from build123d import *

# Parameters (mm, degrees)
BOSS_EXTRUDE1_START = 80.3
BOSS_EXTRUDE1_DEPTH = 2.4
BOSS_EXTRUDE2_START = 80.3
BOSS_EXTRUDE2_DEPTH = 1.6
BOSS_EXTRUDE3_START = 79.3
BOSS_EXTRUDE3_DEPTH = 4.4
BOSS_EXTRUDE4_START = 79.3
SKETCH4_R           = 2.6
BOSS_EXTRUDE4_DEPTH = 4.4
BOSS_EXTRUDE5_START = 82.1
BOSS_EXTRUDE5_DEPTH = 1.6
CHAMFER1_SIZE       = 0.5


with BuildPart() as part:
    # Sketch1 → Boss-Extrude1 (new body)
    with BuildSketch(Plane.XY.offset(BOSS_EXTRUDE1_START)):
        with BuildLine():
            Line((-6, 29), (6, 29))
            ThreePointArc((6, 29), (9.535533906, 30.464466094), (11, 34))
            Line((11, 34), (11, 45))
            ThreePointArc((11, 45), (9.535533906, 48.535533906), (6, 50))
            Line((6, 50), (-6, 50))
            ThreePointArc((-6, 50), (-9.535533906, 48.535533906), (-11, 45))
            Line((-11, 45), (-11, 34))
            ThreePointArc((-11, 34), (-9.535533906, 30.464466094), (-6, 29))
        make_face()
    extrude(amount=BOSS_EXTRUDE1_DEPTH)

    # Sketch2 → Boss-Extrude2 (add)
    with BuildSketch(Plane.XY.offset(BOSS_EXTRUDE2_START)):
        with BuildLine():
            Line((4.5, 53.5), (4.5, 54.7))
            ThreePointArc((4.5, 54.7), (3.181980515, 57.881980515), (0, 59.2))
            ThreePointArc((0, 59.2), (-3.181980515, 57.881980515), (-4.5, 54.7))
            Line((-4.5, 54.7), (-4.5, 53.5))
            ThreePointArc((-4.5, 53.5), (-3.181980515, 50.318019485), (0, 49))
            ThreePointArc((0, 49), (3.181980515, 50.318019485), (4.5, 53.5))
        make_face()
    extrude(amount=BOSS_EXTRUDE2_DEPTH)


with BuildPart() as body_2:
    # Sketch3 → Boss-Extrude3 (new body)
    with BuildSketch(Plane.XY.offset(BOSS_EXTRUDE3_START)):
        with BuildLine():
            Line((-1.8, 56), (-1.8, 53.6))
            ThreePointArc((-1.8, 53.6), (0, 51.8), (1.8, 53.6))
            Line((1.8, 53.6), (1.8, 56))
            ThreePointArc((1.8, 56), (0, 57.8), (-1.8, 56))
        make_face()
    extrude(amount=BOSS_EXTRUDE3_DEPTH)


with BuildPart() as part_1:
    add(part.part)

    # Combine1: cut body 2
    add(body_2.part, mode=Mode.SUBTRACT)


with BuildPart() as body_2_2:
    # Sketch4 → Boss-Extrude4 (new body)
    with BuildSketch(Plane.XY.offset(BOSS_EXTRUDE4_START)):
        with Locations((0, 53.6)):
            Circle(SKETCH4_R)
    extrude(amount=BOSS_EXTRUDE4_DEPTH)


with BuildPart() as part_2:
    add(part_1.part)

    # Combine2: cut body 2 2
    add(body_2_2.part, mode=Mode.SUBTRACT)


with BuildPart() as body_2_3:
    # Sketch5 → Boss-Extrude5 (new body)
    with BuildSketch(Plane.XY.offset(BOSS_EXTRUDE5_START)):
        with BuildLine():
            Line((-5.5, 31.5), (5.5, 31.5))
            ThreePointArc((5.5, 31.5), (7.621320344, 32.378679656), (8.5, 34.5))
            Line((8.5, 34.5), (8.5, 44.5))
            ThreePointArc((8.5, 44.5), (7.621320344, 46.621320344), (5.5, 47.5))
            Line((5.5, 47.5), (-5.5, 47.5))
            ThreePointArc((-5.5, 47.5), (-7.621320344, 46.621320344), (-8.5, 44.5))
            Line((-8.5, 44.5), (-8.5, 34.5))
            ThreePointArc((-8.5, 34.5), (-7.621320344, 32.378679656), (-5.5, 31.5))
        make_face()
    extrude(amount=BOSS_EXTRUDE5_DEPTH)


with BuildPart() as part_3:
    add(part_2.part)

    # Combine3: cut body 2 3
    add(body_2_3.part, mode=Mode.SUBTRACT)

    # Chamfer1
    chamfer1_edges = [part_3.edges().sort_by_distance(p)[0] for p in [
        (9.535533906, 30.464466094, 82.7),
        (11, 39.5, 82.7),
        (9.535533906, 48.535533906, 82.7),
        (0, 50, 82.7),
        (-9.535533906, 48.535533906, 82.7),
        (-11, 39.5, 82.7),
        (-9.535533906, 30.464466094, 82.7),
        (0, 29, 82.7),
    ]]
    chamfer(chamfer1_edges, length=CHAMFER1_SIZE)


solid = part_3.part
For this review, take the finished solid that the model builds, in its own axes (mm). A direction names the side the tool comes from. Round coordinates to 2 decimals unless told otherwise and drop trailing zeros. Write each loop counter-clockwise with the first axis right and the second up, starting at its lowest first coordinate (ties: lowest second). Pieces come first, ordered by that corner, then holes. Notation, with made-up numbers: (45.5, 30.5) - (104.5, 30.5) arc R24 cw to (104.5, 65.5) - close; hole circle Ø10 at (-2, 86.5). An arc over 180 degrees is marked (long way). Write item = value, one per line. Start each with the question number.
1. For faces 1 (the face through (2, 56, 81.9)), 2 (the face through (7.6, 32.36, 82.4)), 3 (the face through (0, 57.8, 81.1)), list the 3-axis set-ups (+Z, -Z, +X, -X, +Y, -Y) from which the entire face can be reached by the end or side of a thin tool; tool diameter is ignored.
2. Wall thickness on L1, parallel to X at y = 53.6, z = 80.8; L2, parallel to Y at x = 0, z = 80.85; L3, parallel to Y at x = -1, z = 82.15: over which ranges is each line inside the solid? List them lowest first.
3. For pin 1 Ø4 at (x, y) = (5, 41) entering from +Z; pin 2 Ø0.5 at (y, z) = (41.5, 82.5) entering from +X; pin 3 Ø8.5 at (x, y) = (0, 53.6) entering from -Z; pin 4 Ø0.6 at (y, z) = (55.5, 81) entering from +X, all flat-tipped, find the tip position at first contact; note any pin that passes through.
4. Consider section D-D on x = 3.75. State the section outline as (y, z) points.
5. Consider section C-C on x = -2.25. State the section outline as (y, z) points, plus the area to 3 significant figures.
6. Consider section B-B on z = 80.8. State the section outline as (x, y) points.
7. Draft analysis for pull direction Y (two halves, no side actions). For faces 4 (the face through (4.05, 51.54, 81.09)), 5 (the face through (9, 30, 81)), 6 (the face through (-9, 49, 81)), state which applies: released by +Y, released by -Y, zero draft, split by the parting line, or undercut.
8. Consider section A-A on y = 38.5. State the section outline as (x, z) points, plus the area to 4 significant figures.
Evaluation:
q1.face_1 = +Z, +X, -X, +Y
q1.face_2 = +Z
q1.face_3 = +Z, -Z
q2.L1 = -4.5 to -2.6, 2.6 to 4.5
q2.L2 = 29 to 51, 57.8 to 59.2
q2.L3 = 29 to 31.5, 47.5 to 50
q3.pin_1 = 82.1
q3.pin_2 = 10.95
q3.pin_3 = 80.3
q3.pin_4 = 4.47
q4.outline = (29, 80.3) - (50, 80.3) - (50, 82.2) - (49.5, 82.7) - (47.5, 82.7) - (47.5, 82.1) - (31.5, 82.1) - (31.5, 82.7) - (29.5, 82.7) - (29, 82.2) - close; (51.01, 80.3) - (57.19, 80.3) - (57.19, 81.9) - (51.01, 81.9) - close
q5.outline = (29, 80.3) - (52.3, 80.3) - (52.3, 81.9) - (50, 81.9) - (50, 82.2) - (49.5, 82.7) - (47.5, 82.7) - (47.5, 82.1) - (31.5, 82.1) - (31.5, 82.7) - (29.5, 82.7) - (29, 82.2) - close; (54.9, 80.3) - (58.6, 80.3) - (58.6, 81.9) - (54.9, 81.9) - close
q5.area = 50.1 mm2
q6.outline = (-11, 34) arc R5 ccw to (-6, 29) - (6, 29) arc R5 ccw to (11, 34) - (11, 45) arc R5 ccw to (6, 50) - (2.83, 50) arc R4.5 ccw to (4.5, 53.5) - (4.5, 54.7) arc R4.5 ccw to (-4.5, 54.7) - (-4.5, 53.5) arc R4.5 ccw to (-2.83, 50) - (-6, 50) arc R5 ccw to (-11, 45) - close; hole (-1.8, 55.48) arc R2.6 ccw (long way) to (1.8, 55.48) - (1.8, 56) arc R1.8 ccw to (-1.8, 56) - close
q7.face_4 = undercut
q7.face_5 = released by -Y
q7.face_6 = released by +Y
q8.outline = (-11, 80.3) - (11, 80.3) - (11, 82.2) - (10.5, 82.7) - (8.5, 82.7) - (8.5, 82.1) - (-8.5, 82.1) - (-8.5, 82.7) - (-10.5, 82.7) - (-11, 82.2) - close
q8.area = 42.35 mm2
